```python
from build123d import *

# Parameters (mm, degrees)
SKETCH1_W           = 25.4
SKETCH1_H           = 12.7
BOSS_EXTRUDE1_DEPTH = 9.9822
SKETCH3_R           = 1.5875
BOSS_EXTRUDE2_DEPTH = 9.525


with BuildPart() as part:
    # Sketch1 → Boss-Extrude1 (new body)
    with BuildSketch(Plane(origin=(0, 0, 0), x_dir=(1, 0, 0), z_dir=(0, 1, 0))):
        with Locations((12.7, 6.35)):
            Rectangle(SKETCH1_W, SKETCH1_H)
    extrude(amount=BOSS_EXTRUDE1_DEPTH)

    # Sketch3 → Boss-Extrude2 (add)
    with BuildSketch(Plane.ZY):
        with Locations((-6.35, 4.9911)):
            Circle(SKETCH3_R)
    extrude(amount=BOSS_EXTRUDE2_DEPTH)


solid = part.part
```
Model file for the job. Use its own axes, mm. A direction names the side the tool comes from. Coordinates: 2 decimals unless noted, no trailing zeros. Order: outer loops, then holes, each group sorted by start corner. A loop starts at its lowest first (then second) coordinate and runs counter-clockwise, first axis right, second up. Notation, with made-up numbers: (-19.75, 86.5) - (-5.75, 86.5) arc R26 ccw to (-5.75, 101.5) - close; hole circle Ø6 at (-12, 72). An arc over 180 degrees is marked (long way). Return JSON: item names as keys, results as strings. Group by question number.
1) Saw through at A-A, the plane z = -6.35. Write the cut outline in (x, y) (3 decimals).
2) Probe line 1 (X direction, y = 7.25, z = -5); line 2 (Z direction, x = -1, y = 4.25). List the from-to ranges inside material, lowest first. Write a range as from..to.
3) Tool access for faces 1 (the cylindrical face through (-4.7, 3.58, -5.62)), 2 (the flat face through (13, 5, -12.7)): list every direction of +Z, -Z, +X, -X, +Y, -Y with a clear straight run to the whole face (end or side of a thin tool).
4) Saw through at D-D, the plane z = -2. Write the cut outline in (x, y), plus the area to 3 significant figures.
5) Saw through at B-B, the plane y = 4.5. Write the cut outline in (x, z) (3 decimals), plus the area to 3 significant figures.
Values found:
{
 "1": {"outline": "(-9.525, 3.404) - (0, 3.404) - (0, 0) - (25.4, 0) - (25.4, 9.982) - (0, 9.982) - (0, 6.579) - (-9.525, 6.579) - close"},
 "2": {"line 1": "x = 0..25.4", "line 2": "z = -7.75..-4.95"},
 "3": {"face 1": "-X", "face 2": "-Z, +X, -X, +Y, -Y"},
 "4": {"outline": "(0, 0) - (25.4, 0) - (25.4, 9.98) - (0, 9.98) - close", "area": "254 mm²"},
 "5": {"outline": "(-9.525, -7.86) - (0, -7.86) - (0, -12.7) - (25.4, -12.7) - (25.4, 0) - (0, 0) - (0, -4.84) - (-9.525, -4.84) - close", "area": "351 mm²"}
}
